```python
from build123d import *

# Parameters (mm, degrees)
SKETCH1_W           = 67.3
SKETCH1_H           = 42.3
SKETCH1_R           = 1.5
SKETCH1_R_2         = 12.5
SKETCH1_R_3         = 2.5
BOSS_EXTRUDE1_DEPTH = 3.175


with BuildPart() as part:
    # Sketch1 → Boss-Extrude1 (new, symmetric)
    with BuildSketch(Plane(origin=(0, 0, 0), x_dir=(1, 0, 0), z_dir=(0, 1, 0))):
        with Locations((-12.5, 0)):
            Rectangle(SKETCH1_W, SKETCH1_H)
        with Locations(Location((15.5, -15.5, 0), (0, 0, 270))):
            Circle(SKETCH1_R, mode=Mode.SUBTRACT)
        with Locations(Location((15.5, 15.5, 0), (0, 0, 270))):
            Circle(SKETCH1_R, mode=Mode.SUBTRACT)
        with Locations(Location((-15.5, 15.5, 0), (0, 0, 270))):
            Circle(SKETCH1_R, mode=Mode.SUBTRACT)
        with Locations(Location((-15.5, -15.5, 0), (0, 0, 270))):
            Circle(SKETCH1_R, mode=Mode.SUBTRACT)
        with Locations(Location((0, 0, 0), (0, 0, 270))):
            Circle(SKETCH1_R_2, mode=Mode.SUBTRACT)
        with Locations(Location((-33.65, 8.65, 0), (0, 0, 270))):
            Circle(SKETCH1_R_3, mode=Mode.SUBTRACT)
        with Locations(Location((-33.65, -8.65, 0), (0, 0, 270))):
            Circle(SKETCH1_R_3, mode=Mode.SUBTRACT)
    extrude(amount=BOSS_EXTRUDE1_DEPTH, both=True)


solid = part.part
```
The listing builds one solid part. Answer for the finished solid, in the listing's coordinates (mm). Round coordinates to 2 decimals unless told otherwise and drop trailing zeros. Loops run counter-clockwise (first coordinate to the right, second up) from the corner with the lowest first, then second, coordinate; pieces in that order, holes last. Notation, with made-up numbers: (-31, 24) - (-23, 24) arc R16 cw to (-23, 48) - close; hole circle Ø7 at (-19, -3.75). An arc over 180 degrees is marked (long way). Use one line per item in the form item = value. Start each with the question number.
1. For a pull along X with two mould halves and no side action, classify faces 1 (the face through (-46.15, 0, 0)), 2 (the face through (-36.09, -0.04, -9.19)), 3 (the face through (-15.43, -0.04, 14)), 4 (the face through (-13, 0, -21.15)) as pulls with the +X half, pulls with the -X half, needs draft (parallel to the pull), parting line crosses it, or undercut.
2. The part is cut by section B-B on z = 15.5. Determine the outline of the cut face in (x, y) (3 decimals).
3. Consider line 1 (X direction, y = -1.25, z = 15.5); line 2 (Z direction, x = 16, y = 2.25); line 3 (X direction, y = 1.75, z = 7.5). Determine where each line is inside the solid, lowest interval first. Write a range as [from, to].
4. The part is cut by section A-A on x = -33.65. Determine the outline of the cut face in (y, z) (3 decimals).
5. Given pin 1 Ø5 at (x, z) = (15.5, 15.5) entering from -Y (3 decimals), flat-ended and moving along its own axis, determine where the tip first touches the part or whether it passes through.
6. The part is cut by section C-C on y = 0. Determine the outline of the cut face in (x, z), then the cut area to 3 significant figures.
7. The part is cut by section D-D on z = 0. Determine the outline of the cut face in (x, y) (3 decimals).
Geometry check:
q1.face_1 = pulls with the -X half
q1.face_2 = undercut
q1.face_3 = undercut
q1.face_4 = needs draft
q2.outline = (-46.15, -3.175) - (-17, -3.175) - (-17, 3.175) - (-46.15, 3.175) - close; (-14, -3.175) - (14, -3.175) - (14, 3.175) - (-14, 3.175) - close; (17, -3.175) - (21.15, -3.175) - (21.15, 3.175) - (17, 3.175) - close
q3.line_1 = [-46.15, -17], [-14, 14], [17, 21.15]
q3.line_2 = [-21.15, -16.91], [-14.09, 14.09], [16.91, 21.15]
q3.line_3 = [-46.15, -35.87], [-31.43, -10], [10, 21.15]
q4.outline = (-3.175, -21.15) - (3.175, -21.15) - (3.175, -11.15) - (-3.175, -11.15) - close; (-3.175, -6.15) - (3.175, -6.15) - (3.175, 6.15) - (-3.175, 6.15) - close; (-3.175, 11.15) - (3.175, 11.15) - (3.175, 21.15) - (-3.175, 21.15) - close
q5.pin_1 = -3.175
q6.outline = (-46.15, -21.15) - (21.15, -21.15) - (21.15, 21.15) - (-46.15, 21.15) - close; hole circle Ø5 at (-33.65, -8.65); hole circle Ø5 at (-33.65, 8.65); hole circle Ø3 at (-15.5, -15.5); hole circle Ø3 at (-15.5, 15.5); hole circle Ø25 at (0, 0); hole circle Ø3 at (15.5, -15.5); hole circle Ø3 at (15.5, 15.5)
q6.area = 2,290 mm^2
q7.outline = (-46.15, -3.175) - (-12.5, -3.175) - (-12.5, 3.175) - (-46.15, 3.175) - close; (12.5, -3.175) - (21.15, -3.175) - (21.15, 3.175) - (12.5, 3.175) - close
